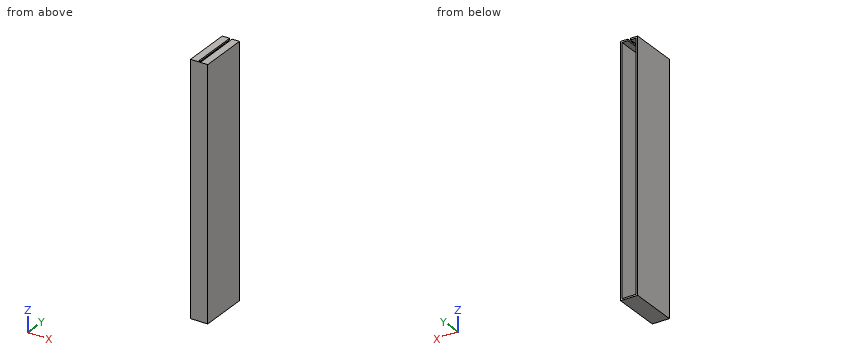
Autodesk Inventor part; units mm, degrees
ref_plane "YZ Plane" through (0, 0, 0) normal (1, 0, 0) x (0, 1, 0)
ref_plane "XZ Plane" through (0, 0, 0) normal (0, 1, 0) x (-1, 0, 0)
ref_plane "XY Plane" through (0, 0, 0) normal (0, 0, 1) x (1, 0, 0)
sketch "Sketch1" plane through (0, 0, 0) normal (0, 1, 0) x (-1, 0, 0)
  line L0 (0, 0) -> (17.9705, 0)
  line L1 (17.9705, 0) -> (17.9705, -259.2705)
  line L2 (17.9705, -259.2705) -> (0, -259.2705)
  line L3 (0, -259.2705) -> (0, 0)
  dimension "d0" = 17.9705
  dimension "d1" = 259.2705
extrude "Extrusion1" add sketch "Sketch1" along normal blind 50.8
shell "Shell1" thickness 1.5875 removed faces 1 at (-5.9902, 50.8, -172.847)
sketch "Sketch2" plane through (-17.9705, 0, 0) normal (0, 0, 1) x (1, 0, 0)
  line L0 (17.9705, 50.8) -> (0, 50.8)
  line L1 (1.5875, 1.5875) -> (16.383, 1.5875)
  line L2 (1.5875, 50.8) -> (16.383, 50.8)
  line L3 (16.383, 50.8) -> (16.383, 1.5875)
  line L4 (16.383, 1.5875) -> (1.5875, 1.5875)
  line L5 (1.5875, 1.5875) -> (1.5875, 50.8)
  line L6 (1.5875, 1.5875) -> (1.5875, 50.8)
  line L7 (7.6835, 50.8) -> (7.6835, 1.5875)
  line L8 (10.287, 50.8) -> (10.287, 1.5875)
  point P0 (17.9705, 0)
  point P1 (10.287, 1.5875)
  point P2 (7.6835, 1.5875)
  dimension "d5" = 0
  dimension "d6" = 6.096
  dimension "d7" = 6.096
extrude "Extrusion2" cut sketch "Sketch2" against normal blind 1.5875 contours L8 L1 L7 L0
properties part number "Wall Lift Test Case"
Source: CAD feature listing. Evaluate the final solid. Frame: model axes, mm. Round coordinates to 2 decimals unless told otherwise and drop trailing zeros. Loops run counter-clockwise (first coordinate to the right, second up) from the corner with the lowest first, then second, coordinate; pieces in that order, holes last.
Q1. First-contact query: P1, Ø2, axis at x = -9.5, z = -233, coming from the -Y side; P2, Ø4.5, axis at x = -12, z = -147.5, coming from the +Y side. Flat tips, straight axial feed; report the tip coordinate or a pass-through.
Q2. Ray query, line 1 (X direction, y = 47.5, z = -124.5); line 2 (Z direction, x = -15.75, y = 25); line 3 (Y direction, x = -12.25, z = -224). Return the intervals inside material, ascending.
Q3. Section B-B, the plane y = 15.5. Return loops of the section in (x, z).
Q4. Section A-A, the plane z = -105. Return loops of the section in (x, y).
Solutions:
1. P1: stops at y = 0
1. P2: stops at y = 1.59
2. line 1: x = -17.97 to -16.38, -1.59 to 0
2. line 2: z = -259.27 to -257.68, -1.59 to 0
2. line 3: y = 0 to 1.59
3. outline: (-17.97, -259.27) - (0, -259.27) - (0, 0) - (-7.68, 0) - (-7.68, -1.59) - (-1.59, -1.59) - (-1.59, -257.68) - (-16.38, -257.68) - (-16.38, -1.59) - (-10.29, -1.59) - (-10.29, 0) - (-17.97, 0) - close
4. outline: (-17.97, 0) - (0, 0) - (0, 50.8) - (-1.59, 50.8) - (-1.59, 1.59) - (-16.38, 1.59) - (-16.38, 50.8) - (-17.97, 50.8) - close
